Read the model definition and answer for the solid it produces. Units are mm, in the model's axes. A direction names the side the tool comes from. Coordinates: 2 decimals unless noted, no trailing zeros. Loops run counter-clockwise (first coordinate to the right, second up) from the corner with the lowest first, then second, coordinate; pieces in that order, holes last. Notation, with made-up numbers: (-31.5, 15) - (19.5, 15) arc R14 ccw to (19.5, 29) - close; hole circle Ø9 at (-40, 57). An arc over 180 degrees is marked (long way). Use one line per item in the form item = value. Start each with the question number.
1) The mould has two halves that part along Z. Classify faces 1 (the face through (153, 1, 87.5)), 2 (the face through (178.901, 1.479, 75.516)), 3 (the face through (159, 3, -1)): released by +Z, released by -Z, zero draft, split by the parting line, or undercut.
2) Which of the six approach directions +Z, -Z, +X, -X, +Y, -Y give full straight-line access (tool end or side, diameter ignored) to faces 4 (the face through (170.54, 1.52, 67.42)), 5 (the face through (159, 0, -1))?
3) Consider line 1 (Z direction, x = 172.5, y = 2.7); line 2 (X direction, y = 2, z = 77.5); line 3 (Z direction, x = 142, y = 2.85). Determine where each line is inside the solid, lowest interval first.
4) This flat-tipped pin is pushed along its axis until it touches: P1, Ø4.5, axis at x = 180.42, z = 77.5, coming from the +Y side. Where does it stop, or does it pass through?
5) A cutting plane is placed at B-B (z = -72.5). Give the vertices of the cut face in (x, y).
6) A cutting plane is placed at A-A (y = 2.15). Give the vertices of the cut face in (x, z), and give its area (3 significant figures).
from build123d import *

# Parameters (mm, degrees)
ESQUISSE1_R             = 2.5
BOSS_EXTRU_1_DEPTH      = 3
ENL_V_MAT_EXTRU_1_DEPTH = 210.585226303


with BuildPart() as part:
    # Esquisse1 → Boss.-Extru.1 (new body)
    with BuildSketch(Plane(origin=(0, 0, 0), x_dir=(1, 0, 0), z_dir=(0, 1, 0))):
        with BuildLine():
            Line((125.70871342, 87.5), (180.42247001, 87.5))
            Line((180.42247001, 87.5), (190.42247001, 87.5))
            Line((190.42247001, 87.5), (190.42247001, 77.5))
            Line((190.42247001, 77.5), (190.42247001, -77.5))
            ThreePointArc((190.42247001, -77.5), (187.493537821, -84.571067812), (180.42247001, -87.5))
            Line((180.42247001, -87.5), (125.70871342, -87.5))
            Line((125.70871342, -87.5), (125.70871342, 87.5))
        make_face()
        with Locations(Location((180.42247001, 77.5, 0), (0, 0, 270))):
            Circle(ESQUISSE1_R, mode=Mode.SUBTRACT)
        with Locations(Location((180.42247001, -77.5, 0), (0, 0, 270))):
            Circle(ESQUISSE1_R, mode=Mode.SUBTRACT)
    extrude(amount=BOSS_EXTRU_1_DEPTH)

    # Esquisse2 → Enlèv. mat.-Extru.1 (cut, through all)
    with BuildSketch(Plane(origin=(0, 3, 0), x_dir=(1, 0, 0), z_dir=(0, 1, 0))):
        with BuildLine():
            Line((138.620155232, -78.124092094), (181.046562103, -35.697685223))
            ThreePointArc((181.046562103, -35.697685223), (181.046562103, -32.162151317), (177.511028197, -32.162151317))
            Line((177.511028197, -32.162151317), (135.084621326, -74.588558188))
            ThreePointArc((135.084621326, -74.588558188), (135.084621326, -78.124092094), (138.620155232, -78.124092094))
        make_face()
        with BuildLine():
            Line((166.90442648, -78.124092094), (181.046562103, -63.98195647))
            ThreePointArc((181.046562103, -63.98195647), (181.046562103, -60.446422564), (177.511028197, -60.446422564))
            Line((177.511028197, -60.446422564), (163.368892574, -74.588558188))
            ThreePointArc((163.368892574, -74.588558188), (163.368892574, -78.124092094), (166.90442648, -78.124092094))
        make_face()
        with BuildLine():
            Line((138.620155232, -49.839820846), (152.762290856, -35.697685223))
            ThreePointArc((152.762290856, -35.697685223), (152.762290856, -32.162151317), (149.22675695, -32.162151317))
            Line((149.22675695, -32.162151317), (135.084621326, -46.30428694))
            ThreePointArc((135.084621326, -46.30428694), (135.084621326, -49.839820846), (138.620155232, -49.839820846))
        make_face()
        with BuildLine():
            Line((135.084621326, 74.588558188), (177.511028197, 32.162151317))
            ThreePointArc((177.511028197, 32.162151317), (181.046562103, 32.162151317), (181.046562103, 35.697685223))
            Line((181.046562103, 35.697685223), (138.620155232, 78.124092094))
            ThreePointArc((138.620155232, 78.124092094), (135.084621326, 78.124092094), (135.084621326, 74.588558188))
        make_face()
        with BuildLine():
            Line((135.084621326, 46.30428694), (149.22675695, 32.162151317))
            ThreePointArc((149.22675695, 32.162151317), (152.762290856, 32.162151317), (152.762290856, 35.697685223))
            Line((152.762290856, 35.697685223), (138.620155232, 49.839820846))
            ThreePointArc((138.620155232, 49.839820846), (135.084621326, 49.839820846), (135.084621326, 46.30428694))
        make_face()
    extrude(amount=-ENL_V_MAT_EXTRU_1_DEPTH, mode=Mode.SUBTRACT)


solid = part.part
Found:
q1.face_1 = released by +Z
q1.face_2 = undercut
q1.face_3 = zero draft
q2.face_4 = +Y, -Y
q2.face_5 = +Z, -Z, +X, -X, -Y
q3.line_1 = -87.5 to -44.24, -37.17 to 37.17, 44.24 to 65.46, 72.53 to 87.5
q3.line_2 = 125.71 to 134.63, 139.24 to 162.91, 167.53 to 177.92, 182.92 to 190.42
q3.line_3 = -87.5 to -74.74, -67.67 to -46.46, -39.39 to 39.39, 46.46 to 67.67, 74.74 to 87.5
q4.P1 = through
q5.outline = (125.71, 0) - (137.17, 0) - (137.17, 3) - (125.71, 3) - close; (144.24, 0) - (190.42, 0) - (190.42, 3) - (144.24, 3) - close
q6.outline = (125.71, -87.5) - (190.42, -87.5) - (190.42, 77.5) arc R10 ccw to (180.42, 87.5) - (125.71, 87.5) - close; hole (135.08, -74.59) arc R2.5 ccw to (138.62, -78.12) - (181.05, -35.7) arc R2.5 ccw to (177.51, -32.16) - close; hole (135.08, -46.3) arc R2.5 ccw to (138.62, -49.84) - (152.76, -35.7) arc R2.5 ccw to (149.23, -32.16) - close; hole (135.08, 46.3) - (149.23, 32.16) arc R2.5 ccw to (152.76, 35.7) - (138.62, 49.84) arc R2.5 ccw to start; hole (135.08, 74.59) - (177.51, 32.16) arc R2.5 ccw to (181.05, 35.7) - (138.62, 78.12) arc R2.5 ccw to start; hole (163.37, 74.59) - (177.51, 60.45) arc R2.5 ccw to (181.05, 63.98) - (166.9, 78.12) arc R2.5 ccw to start; hole circle Ø5 at (180.42, -77.5); hole circle Ø5 at (180.42, 77.5)
q6.area = 10,300 mm^2
